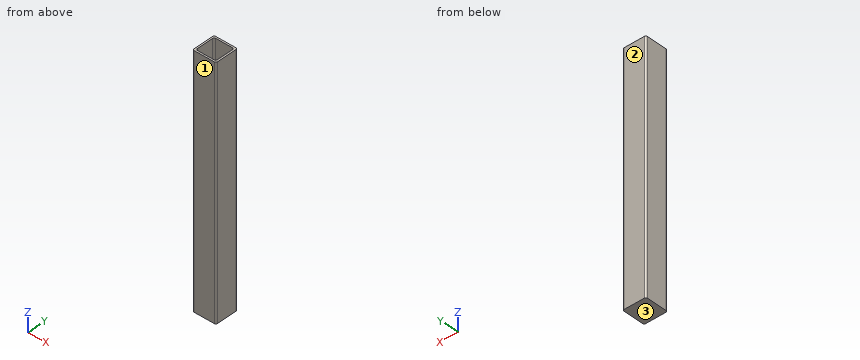
from build123d import *

# Parameters (mm, degrees)
BOSS_EXTRUDE1_DEPTH = 397
BOSS_EXTRUDE2_START = 0.678713738
BOSS_EXTRUDE2_DEPTH = 0.678713738


with BuildPart() as part:
    # Sketch1 → Boss-Extrude1 (new body)
    with BuildSketch(Plane.XY):
        with BuildLine():
            Line((2.54, 0), (35.56, 0))
            ThreePointArc((35.56, 0), (37.356051224, -0.743948776), (38.1, -2.54))
            Line((38.1, -2.54), (38.1, -35.56))
            ThreePointArc((38.1, -35.56), (37.356051224, -37.356051224), (35.56, -38.1))
            Line((35.56, -38.1), (2.54, -38.1))
            ThreePointArc((2.54, -38.1), (0.743948776, -37.356051224), (0, -35.56))
            Line((0, -35.56), (0, -2.54))
            ThreePointArc((0, -2.54), (0.743948776, -0.743948776), (2.54, 0))
        make_face()
        with BuildLine():
            Line((5.3086, -2.7686), (32.7914, -2.7686))
            ThreePointArc((32.7914, -2.7686), (34.587451224, -3.512548776), (35.3314, -5.3086))
            Line((35.3314, -5.3086), (35.3314, -32.7914))
            ThreePointArc((35.3314, -32.7914), (34.587451224, -34.587451224), (32.7914, -35.3314))
            Line((32.7914, -35.3314), (5.3086, -35.3314))
            ThreePointArc((5.3086, -35.3314), (3.512548776, -34.587451224), (2.7686, -32.7914))
            Line((2.7686, -32.7914), (2.7686, -5.3086))
            ThreePointArc((2.7686, -5.3086), (3.512548776, -3.512548776), (5.3086, -2.7686))
        make_face(mode=Mode.SUBTRACT)
    extrude(amount=BOSS_EXTRUDE1_DEPTH)

    # Sketch2 → Boss-Extrude2 (add)
    with BuildSketch(Plane(origin=(0, 0, 0), x_dir=(-1, 0, 0), z_dir=(0, 0, -1)).offset(BOSS_EXTRUDE2_START)):
        with BuildLine():
            Line((0, -35.56), (0, -2.54))
            ThreePointArc((0, -2.54), (-0.743948776, -0.743948776), (-2.54, 0))
            Line((-2.54, 0), (-35.56, 0))
            ThreePointArc((-35.56, 0), (-37.356051224, -0.743948776), (-38.1, -2.54))
            Line((-38.1, -2.54), (-38.1, -35.56))
            ThreePointArc((-38.1, -35.56), (-37.356051224, -37.356051224), (-35.56, -38.1))
            Line((-35.56, -38.1), (-2.54, -38.1))
            ThreePointArc((-2.54, -38.1), (-0.743948776, -37.356051224), (0, -35.56))
        make_face()
    extrude(amount=-BOSS_EXTRUDE2_DEPTH)


solid = part.part
Input: part model. Units: mm. Frame: model coordinates. Face numbers are marked on the shaded views. Give positions to 0.01 mm unless a question says otherwise; leave off trailing zeros. Loops run counter-clockwise (first coordinate to the right, second up) from the corner with the lowest first, then second, coordinate; pieces in that order, holes last. Notation, with made-up numbers: M 40,27.5 L 71,27.5 A8 cw 71,31.5 Z; hole C -37,69 d11. An arc over 180 degrees is marked long. Use CSV: the item, a comma, the result in double quotes.
(1) Section B-B, the plane y = -28. Return loops of the section in (x, z).
Outcome:
outline,"M 0,-0.68 L 38.1,-0.68 L 38.1,397 L 35.33,397 L 35.33,0 L 2.77,0 L 2.77,397 L 0,397 Z"
(2) Material intervals for L1, parallel to Y at x = 22, z = 318.5; L2, parallel to X at y = -30, z = 26.5; L3, parallel to X at y = -2, z = 251, sorted ascending. Write a range as [from, to].
Outcome:
L1,"y = [-38.1, -35.33], [-2.77, 0]"
L2,"x = [0, 2.77], [35.33, 38.1]"
L3,"x = [0.06, 38.04]"
(3) Section A-A, the plane z = 364.5. Return loops of the section in (x, y), plus the area to 3 significant figures.
Outcome:
outline,"M 0,-35.56 A2.54 ccw 2.54,-38.1 L 35.56,-38.1 A2.54 ccw 38.1,-35.56 L 38.1,-2.54 A2.54 ccw 35.56,0 L 2.54,0 A2.54 ccw 0,-2.54 Z; hole M 2.77,-32.79 A2.54 ccw 5.31,-35.33 L 32.79,-35.33 A2.54 ccw 35.33,-32.79 L 35.33,-5.31 A2.54 ccw 32.79,-2.77 L 5.31,-2.77 A2.54 ccw 2.77,-5.31 Z"
area,"391 mm²"
(4) Section C-C, the plane x = 28. Return loops of the section in (y, z), plus the area to 3 significant figures.
Outcome:
outline,"M -38.1,-0.68 L 0,-0.68 L 0,397 L -2.77,397 L -2.77,0 L -35.33,0 L -35.33,397 L -38.1,397 Z"
area,"2,220 mm²"
(5) Pull-direction query (Y, two-part tool) for the marked faces 1, 2 and 3; classes: pulls with the +Y half, pulls with the -Y half, needs draft (parallel to the pull), parting line crosses it, or undercut.
Outcome:
face 1,"pulls with the -Y half"
face 2,"pulls with the +Y half"
face 3,"needs draft"
(6) Pin query (flat end, axial travel): P1, Ø16.5, axis at x = 11.5, y = -13, coming from the +Z side. Return the tip coordinate at first contact, or that it passes through.
Outcome:
P1,"stops at z = 0"
